Autodesk Fusion 360 part; units mm, degrees
sketch "Sketch1" plane through (0, 0, 0) normal (0, 1, 0) x (1, 0, 0)
  circle A0 centre (0, 0) radius 4.2
  circle A1 centre (0, 0) radius 10
  dimension "d1" = 8.4
  dimension "d2" = 20
extrude "Extrude1" add sketch "Sketch1" along normal blind 1.5 makes body 1
copy_body "Body->Comp1" bodies 1 removing the originals makes body 2 in component "M8x20 washer"
component "M8x20 washer" placed x (1, 0, 0) y (0, 1, 0) z (0, 0, 1) at (0, 0, 0)
For this review, take the finished solid that the model builds, in its own axes (mm). Give positions to 0.01 mm unless a question says otherwise; leave off trailing zeros. Loops run counter-clockwise (first coordinate to the right, second up) from the corner with the lowest first, then second, coordinate; pieces in that order, holes last. Notation, with made-up numbers: M 62,53 L 78,53 A16 cw 78,79 Z; hole C -3,79 d9. An arc over 180 degrees is marked long. Put each result on its own line as item: value. Start each with the question number.
(1) Add section D-D, the plane x = 8. Write out the cut boundary in (y, z), then the cut area to 3 significant figures.
(2) The part is to be moulded in two halves that separate along Z. For faces 1 (the cylindrical face through (-2.17, 0.74, -9.76)), 2 (the flat face through (4, 0, 2)), 3 (the cylindrical face through (4.006, 0.74, 1.262)), say which applies: +Z half, -Z half, draft (parallel to the pull), parting line (faces both ways), or undercut.
(3) Add section B-B, the plane z = 0. Write out the cut boundary in (x, y), then the cut area to 3 significant figures.
(4) Add section C-C, the plane y = 1.05. Write out the cut boundary in (x, z), then the cut area to 3 significant figures.
(5) Wall thickness on L1, parallel to Z at x = 0, y = 0.8; L2, parallel to Z at x = 0.75, y = 0.9: over which ranges is each line inside the solid? List them lowest first.
(6) For pin 1 (12 mm diameter, centred on x = 2, z = 1.5, fed in from +Y); pin 2 (5 mm diameter, centred on x = 0, z = 0, fed in from +Y), all flat-tipped, find the tip position at first contact; note any pin that passes through.
(7) Add section A-A, the plane x = 0. Write out the cut boundary in (y, z), then the cut area to 3 significant figures.
Result:
1. outline: M 0,-6 L 1.5,-6 L 1.5,6 L 0,6 Z
1. area: 18.0 mm^2
2. face 1: parting line
2. face 2: draft
2. face 3: undercut
3. outline: M -10,0 L -4.2,0 L -4.2,1.5 L -10,1.5 Z; M 4.2,0 L 10,0 L 10,1.5 L 4.2,1.5 Z
3. area: 17.4 mm^2
4. outline: C 0,0 d20; hole C 0,0 d8.4
4. area: 259 mm^2
5. L1: z = -10 to -4.2, 4.2 to 10
5. L2: z = -9.97 to -4.13, 4.13 to 9.97
6. pin 1: stops at y = 1.5
6. pin 2: passes through
7. outline: M 0,-10 L 1.5,-10 L 1.5,-4.2 L 0,-4.2 Z; M 0,4.2 L 1.5,4.2 L 1.5,10 L 0,10 Z
7. area: 17.4 mm^2
